Build history of the part. All positions in model axes, mm. A direction names the side the tool comes from. Give positions to 0.01 mm unless a question says otherwise; leave off trailing zeros. Order: outer loops, then holes, each group sorted by start corner. A loop starts at its lowest first (then second) coordinate and runs counter-clockwise, first axis right, second up. Notation, with made-up numbers: (4.5, -36.75) -> (47.5, -36.75) arc R17 ccw to (47.5, -24.75) -> close; hole circle Ø1 at (20.5, 60.25). An arc over 180 degrees is marked (long way). One line per question, with ' | ' between items. Start each with the question number.
(1) Cut at A-A (y = -13.75). Give the cut face in (x, z), then the cut area to 3 significant figures.
(2) Which spindle directions (+Z, -Z, +X, -X, +Y, -Y) get a long thin tool onto all of the face, cutting with end or side? Do faces 4 (the face through (-23.589, -21.805, 3.944)), 5 (the face through (-44.443, -20.413, 3.944)). Say none if no direction does.
(3) Drill centre lines: L1, parallel to X at y = -14.25, z = 5.25; L2, parallel to X at y = -14, z = 0.5; L3, parallel to Y at x = -23, z = 2.25. Where is each one in solid material? Low to high. Write a range as from..to.
(4) Pull direction X, two halves, no side cores. Call faces 1 (the face through (-43.353, -12.974, 3.944)), 2 (the face through (-33, -12.589, 4)), 3 (the face through (-22.482, -20.414, 3.944)): +X half, -X half, draft (parallel to the pull), parting line (faces both ways), or undercut.
(5) Cut at C-C (z = 1.25). Give the cut face in (x, y), then the cut area to 3 significant figures.
(6) Cut at B-B (x = -38). Give the cut face in (y, z), then the cut area to 3 significant figures.
(7) Cut at D-D (x = -25). Give the cut face in (y, z), then the cut area to 3 significant figures.
(8) Pin check, flat tip, straight feed: pin 1 Ø1.5 at (y, z) = (-20.5, 1) entering from -X. Stop position of the tip, or through.
from build123d import *

# Parameters (mm, degrees)
EXTRUDE_1_DEPTH = 8
FILLET_1_R      = 0.8


with BuildPart() as part:
    # 草图1 → 凸台-拉伸1 (new body)
    with BuildSketch(Plane.XY):
        with BuildLine():
            Line((-25.471055476, -12.589310126), (-41.471055476, -12.589310126))
            ThreePointArc((-41.471055476, -12.589310126), (-38.076942926, -13.995197576), (-36.671055476, -17.389310126))
            ThreePointArc((-36.671055476, -17.389310126), (-38.076942926, -20.783422675), (-41.471055476, -22.189310126))
            Line((-41.471055476, -22.189310126), (-25.471055476, -22.189310126))
            ThreePointArc((-25.471055476, -22.189310126), (-30.271055476, -17.389310126), (-25.471055476, -12.589310126))
        make_face()
        with BuildLine():
            ThreePointArc((-36.671055476, -17.389310126), (-38.076942926, -13.995197576), (-41.471055476, -12.589310126))
            Line((-41.471055476, -12.589310126), (-41.471055476, -13.389310126))
            ThreePointArc((-41.471055476, -13.389310126), (-38.642628351, -14.560883001), (-37.471055476, -17.389310126))
            ThreePointArc((-37.471055476, -17.389310126), (-38.642628351, -20.21773725), (-41.471055476, -21.389310126))
            Line((-41.471055476, -21.389310126), (-41.471055476, -22.189310126))
            ThreePointArc((-41.471055476, -22.189310126), (-38.076942926, -20.783422675), (-36.671055476, -17.389310126))
        make_face()
        with BuildLine():
            Line((-25.471055476, -13.389310126), (-25.471055476, -12.589310126))
            ThreePointArc((-25.471055476, -12.589310126), (-30.271055476, -17.389310126), (-25.471055476, -22.189310126))
            Line((-25.471055476, -22.189310126), (-25.471055476, -21.389310126))
            ThreePointArc((-25.471055476, -21.389310126), (-29.471055476, -17.389310126), (-25.471055476, -13.389310126))
        make_face()
        with BuildLine():
            ThreePointArc((-21.971055476, -14.104496584), (-23.564108308, -12.984363758), (-25.471055476, -12.589310126))
            Line((-25.471055476, -12.589310126), (-25.471055476, -13.389310126))
            ThreePointArc((-25.471055476, -13.389310126), (-23.43954947, -13.943590557), (-21.971055476, -15.452818452))
            Line((-21.971055476, -15.452818452), (-21.971055476, -14.104496584))
        make_face()
        with BuildLine():
            Line((-25.471055476, -21.389310126), (-25.471055476, -22.189310126))
            ThreePointArc((-25.471055476, -22.189310126), (-23.564108308, -21.794256493), (-21.971055476, -20.674123667))
            Line((-21.971055476, -20.674123667), (-21.971055476, -19.325801799))
            ThreePointArc((-21.971055476, -19.325801799), (-23.43954947, -20.835029694), (-25.471055476, -21.389310126))
        make_face()
        with BuildLine():
            ThreePointArc((-21.971055476, -14.104496584), (-23.564108308, -12.984363758), (-25.471055476, -12.589310126))
            Line((-25.471055476, -12.589310126), (-25.471055476, -13.389310126))
            ThreePointArc((-25.471055476, -13.389310126), (-23.43954947, -13.943590557), (-21.971055476, -15.452818452))
            Line((-21.971055476, -15.452818452), (-21.971055476, -14.104496584))
        make_face()
        with BuildLine():
            Line((-25.471055476, -21.389310126), (-25.471055476, -22.189310126))
            ThreePointArc((-25.471055476, -22.189310126), (-23.564108308, -21.794256493), (-21.971055476, -20.674123667))
            Line((-21.971055476, -20.674123667), (-21.971055476, -19.325801799))
            ThreePointArc((-21.971055476, -19.325801799), (-23.43954947, -20.835029694), (-25.471055476, -21.389310126))
        make_face()
        with BuildLine():
            Line((-41.471055476, -13.389310126), (-41.471055476, -12.589310126))
            ThreePointArc((-41.471055476, -12.589310126), (-43.378002644, -12.984363758), (-44.971055476, -14.104496584))
            Line((-44.971055476, -14.104496584), (-44.971055476, -15.452818452))
            ThreePointArc((-44.971055476, -15.452818452), (-43.502561482, -13.943590557), (-41.471055476, -13.389310126))
        make_face()
        with BuildLine():
            Line((-41.471055476, -22.189310126), (-41.471055476, -21.389310126))
            ThreePointArc((-41.471055476, -21.389310126), (-43.502561482, -20.835029694), (-44.971055476, -19.325801799))
            Line((-44.971055476, -19.325801799), (-44.971055476, -20.674123667))
            ThreePointArc((-44.971055476, -20.674123667), (-43.378002644, -21.794256493), (-41.471055476, -22.189310126))
        make_face()
        with BuildLine():
            Line((-41.471055476, -13.389310126), (-41.471055476, -12.589310126))
            ThreePointArc((-41.471055476, -12.589310126), (-43.378002644, -12.984363758), (-44.971055476, -14.104496584))
            Line((-44.971055476, -14.104496584), (-44.971055476, -15.452818452))
            ThreePointArc((-44.971055476, -15.452818452), (-43.502561482, -13.943590557), (-41.471055476, -13.389310126))
        make_face()
        with BuildLine():
            Line((-41.471055476, -22.189310126), (-41.471055476, -21.389310126))
            ThreePointArc((-41.471055476, -21.389310126), (-43.502561482, -20.835029694), (-44.971055476, -19.325801799))
            Line((-44.971055476, -19.325801799), (-44.971055476, -20.674123667))
            ThreePointArc((-44.971055476, -20.674123667), (-43.378002644, -21.794256493), (-41.471055476, -22.189310126))
        make_face()
    extrude(amount=EXTRUDE_1_DEPTH)

    # 圆角1
    # the kernel refuses this fillet: 0.8 mm, written as the material it takes off along each edge
    with BuildSketch(Plane(origin=(-21.971055476, -15.452818452, -4.122167705), x_dir=(0, 1, 0), z_dir=(0, 0, 1)), Plane(origin=(-44.971055476, -19.325801799, -4.122167705), x_dir=(0, -1, 0), z_dir=(0, 0, 1))) as fillet_1_piece_1:
        with BuildLine():
            CenterArc((1.884003799, 0.594175789), FILLET_1_R, 142.743805491, 85.219808153)
            Line((1.247254554, 1.078479824), (1.234519569, 1.088165905))
            ThreePointArc((1.234519569, 1.088165905), (0.66933609, 0.486377982), (-0.007745967, 0.014))
            Line((-0.007745967, 0.014), (0, -0.016))
            ThreePointArc((0, -0.016), (0.674160934, -0.016), (1.337608229, -0.011883516))
            Line((1.337608229, -0.011883516), (1.348321868, 0))
        make_face()
    extrude(amount=16.24433541, mode=Mode.SUBTRACT)
    with BuildSketch(Plane(origin=(-21.971055476, -19.325801799, -4.122167705), x_dir=(-0.6540732337391989, -0.7564312294623664, 0), z_dir=(0, 0, 1))) as fillet_1_piece_2:
        with BuildLine():
            CenterArc((1.81375379, 0.782823335), FILLET_1_R, 172.885801288, 85.219808153)
            Line((1.019912768, 0.881901244), (1.004035948, 0.883882803))
            ThreePointArc((1.004035948, 0.883882803), (0.499491212, 0.453053522), (-0.010465172, 0.0121029))
            Line((-0.010465172, 0.0121029), (0.003297734, -0.015656467))
            ThreePointArc((0.003297734, -0.015656467), (0.824433541, 0.069883326), (1.645569348, -0.015656467))
            Line((1.645569348, -0.015656467), (1.648867082, 0))
        make_face()
    extrude(amount=16.24433541, mode=Mode.SUBTRACT)
    with BuildSketch(Plane(origin=(-44.971055476, -15.452818452, -4.122167705), x_dir=(0, 1, 0), z_dir=(0, 0, 1))) as fillet_1_piece_3:
        with BuildLine():
            CenterArc((1.884003799, -0.594175789), FILLET_1_R, 132.036386357, 85.219808153)
            Line((1.247254554, -1.078479824), (1.234519569, -1.088165905))
            ThreePointArc((1.234519569, -1.088165905), (0.66933609, -0.486377982), (-0.007745967, -0.014))
            Line((-0.007745967, -0.014), (0, 0.016))
            ThreePointArc((0, 0.016), (0.674160934, 0.016), (1.337608229, 0.011883516))
            Line((1.337608229, 0.011883516), (1.348321868, 0))
        make_face()
    extrude(amount=16.24433541, mode=Mode.SUBTRACT)


solid = part.part
Result set:
1) outline: (-44.6, 0) -> (-43.13, 0) -> (-43.13, 8) -> (-44.6, 8) -> close; (-39.81, 0) -> (-27.13, 0) -> (-27.13, 8) -> (-39.81, 8) -> close; (-23.81, 0) -> (-22.34, 0) -> (-22.34, 8) -> (-23.81, 8) -> close | area: 125 mm2
2) face 4: +Z, -Z, +X, -Y | face 5: +Z, -Z
3) L1: x = -44.8..-43.96, -38.99..-27.95, -22.98..-22.15 | L2: x = -44.87..-43.6, -39.35..-27.6, -23.35..-22.07 | L3: y = -21.5..-20.54, -14.24..-13.27
4) face 1: -X half | face 2: draft | face 3: undercut
5) outline: (-44.97, -20.67) arc R4.8 ccw to (-41.47, -22.19) -> (-25.47, -22.19) arc R4.8 ccw to (-21.97, -20.67) arc R0.8 ccw to (-23.05, -20.57) arc R4 cw (long way) to (-23.05, -14.21) arc R0.8 ccw to (-21.97, -14.1) arc R4.8 ccw to (-25.47, -12.59) -> (-41.47, -12.59) arc R4.8 ccw to (-44.97, -14.1) arc R0.8 ccw to (-43.89, -14.21) arc R4 cw (long way) to (-43.89, -20.57) arc R0.8 ccw to start | area: 114 mm2
6) outline: (-22.19, 0) -> (-19.38, 0) -> (-19.38, 8) -> (-22.19, 8) -> close; (-15.4, 0) -> (-12.59, 0) -> (-12.59, 8) -> (-15.4, 8) -> close | area: 45.0 mm2
7) outline: (-22.17, 0) -> (-21.36, 0) -> (-21.36, 8) -> (-22.17, 8) -> close; (-13.42, 0) -> (-12.61, 0) -> (-12.61, 8) -> (-13.42, 8) -> close | area: 12.9 mm2
8) pin 1: stops at x = -44.97
